Job drawing, mm, ordinate dimensions from the low corner. One solid piece. A direction names the side the tool comes from. Give positions to 0.01 mm unless a question says otherwise; leave off trailing zeros. Loops run counter-clockwise (first coordinate to the right, second up) from the corner with the lowest first, then second, coordinate; pieces in that order, holes last. Notation, with made-up numbers: M 66.25,41.25 L 75.25,41.25 A18 cw 75.25,45.25 Z; hole C 18,50 d2. An arc over 180 degrees is marked long. Answer in a Markdown table with one row per item.
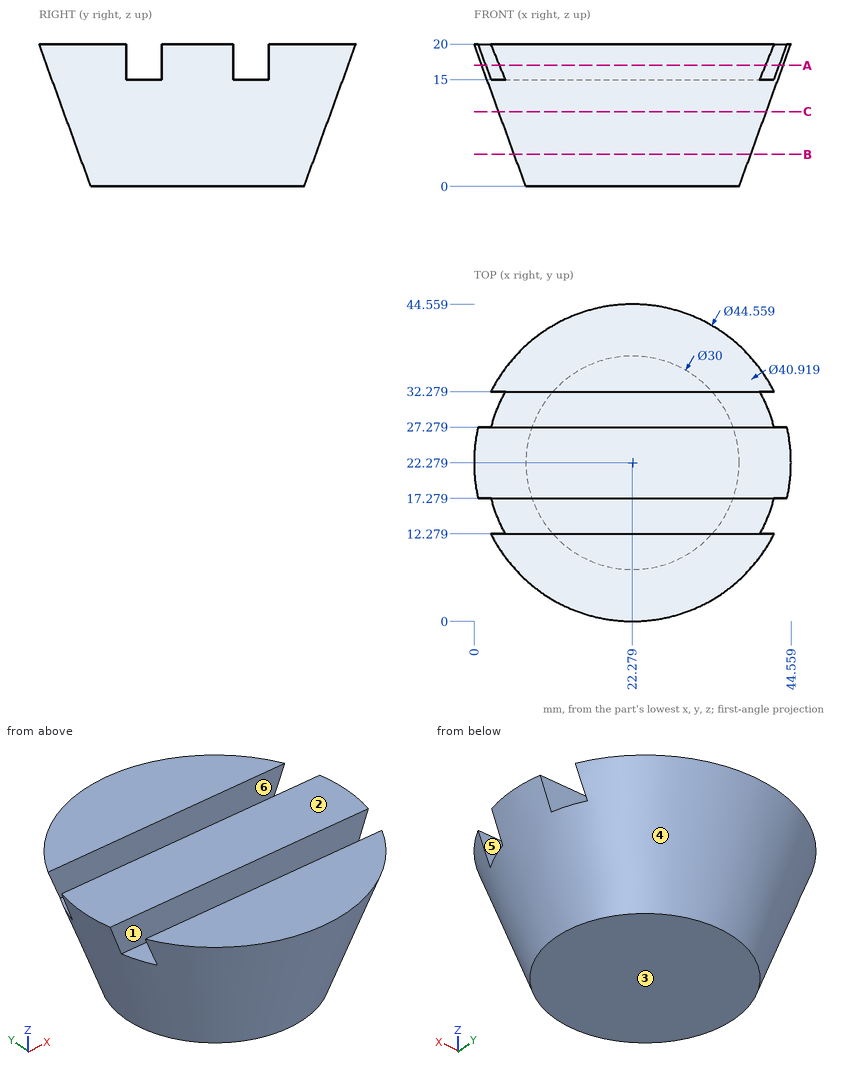
(1) Drill centre lines: line 1 along Y through (x, z) = (25.5, 16.5); line 2 along Y through (x, z) = (42, 18.75); line 3 along Z through (x, y) = (24.5, 28.5). Where is each one in solid material? Low to high.
Recorded:
| item | result |
|---|---|
| line 1 | y = 1.52 to 12.28, 17.28 to 27.28, 32.28 to 43.04 |
| line 2 | y = 17.28 to 27.28 |
| line 3 | z = 0 to 15 |
(2) Which spindle directions (+Z, -Z, +X, -X, +Y, -Y) get a long thin tool onto all of the face, cutting with end or side? Do the marked faces 1 and 2. Say none if no direction does.
Recorded:
| item | result |
|---|---|
| face 1 | +Z, +X, -X |
| face 2 | +Z, +X, -X, +Y, -Y |
(3) Pull direction Y, two halves, no side cores. Call the marked faces 3, 4, 5 and 6: +Y half, -Y half, draft (parallel to the pull), parting line (faces both ways), or undercut.
Recorded:
| item | result |
|---|---|
| face 3 | draft |
| face 4 | parting line |
| face 5 | undercut |
| face 6 | undercut |
(4) Saw through at B-B (z = 4.5). Write the cut outline in (x, y) (1 decimal), plus the area to 3 significant figures.
Recorded:
| item | result |
|---|---|
| outline | C 22.3,22.3 d33.3 |
| area | 870 mm^2 |
(5) Saw through at A-A (z = 17). Write the cut outline in (x, y) (1 decimal), plus the area to 4 significant figures.
Recorded:
| item | result |
|---|---|
| outline | M 1.7,17.3 L 42.9,17.3 A21.2 ccw 42.9,27.3 L 1.7,27.3 A21.2 ccw Z; M 3.6,12.3 A21.2 ccw 41,12.3 Z; M 3.6,32.3 L 41,32.3 A21.2 ccw Z |
| area | 1,015 mm^2 |
(6) Saw through at C-C (z = 10.5). Write the cut outline in (x, y), plus the area to 3 significant figures.
Recorded:
| item | result |
|---|---|
| outline | C 22.28,22.28 d37.64 |
| area | 1,110 mm^2 |
(7) Pin check, flat tips, straight feed: pin 1 Ø1 at (y, z) = (29, 9) entering from -X; pin 2 Ø2 at (y, z) = (7.5, 17.5) entering from +X; pin 3 Ø2.5 at (x, z) = (21.5, 18) entering from -Y (1 decimal). Stop position of each tip, or through.
Recorded:
| item | result |
|---|---|
| pin 1 | stops at x = 5.01 |
| pin 2 | stops at x = 38.74 |
| pin 3 | stops at y = 0.3 |
